from build123d import *

# Parameters (mm, degrees)
F_3_8_0_375_DIAMETER_HOLE1_D     = 9.525
F_3_8_0_375_DIAMETER_HOLE1_DEPTH = 5.999988
F_3_8_0_375_DIAMETER_HOLE1_TIP   = 2.861598698
SKETCH6_W                        = 0.6
SKETCH6_H                        = 2
BOSS_EXTRUDE1_DEPTH              = 5.5


with BuildPart() as part:
    # Sketch1 → Revolve2 (revolve)
    with BuildSketch(Plane(origin=(0, 0, 0), x_dir=(1, 0, 0), z_dir=(0, 1, 0))):
        Polygon((0, 0), (6.35, 0), (6.35, 17.5), (7.5, 17.5), (7.5, 18.5), (6.5, 19.5), (0, 19.5), align=None)
    revolve(axis=Axis((0, 0, -19.5), (0, 0, 1)))

    # 3/8 (0.375) Diameter Hole1
    with Locations(Plane(origin=(0, 0, -19.5), x_dir=(-1, 0, 0), z_dir=(0, 0, -1))):
        with Locations((0, 0)):
            Hole(F_3_8_0_375_DIAMETER_HOLE1_D / 2, depth=F_3_8_0_375_DIAMETER_HOLE1_DEPTH)
            with Locations((0, 0, -(F_3_8_0_375_DIAMETER_HOLE1_DEPTH + F_3_8_0_375_DIAMETER_HOLE1_TIP / 2))):  # 118° drill point
                Cone(0, F_3_8_0_375_DIAMETER_HOLE1_D / 2, F_3_8_0_375_DIAMETER_HOLE1_TIP, mode=Mode.SUBTRACT)

    # Sketch6 → Boss-Extrude1 (add)
    with BuildSketch(Plane.XY):
        with Locations((-3, 0)):
            Rectangle(SKETCH6_W, SKETCH6_H)
    boss_extrude1 = extrude(amount=BOSS_EXTRUDE1_DEPTH)

    # Mirror1: Boss-Extrude1 across plane
    add(boss_extrude1.mirror(Plane(origin=(0, 0, 0), x_dir=(0, 0, 1), z_dir=(1, 0, 0))))


solid = part.part
Verification items for the finished model (mm, model axes). A direction names the side the tool comes from. Coordinates: 2 decimals unless noted, no trailing zeros. Write each loop counter-clockwise with the first axis right and the second up, starting at its lowest first coordinate (ties: lowest second). Pieces come first, ordered by that corner, then holes. Notation, with made-up numbers: M 5,-39 L 51,-39 A20 cw 51,-33 Z; hole C 39,70 d4. An arc over 180 degrees is marked long. One line per question, with ' | ' between items.
1) Release check for a two-part mould opening along X. For faces 4 (the face through (-1.38, -6.2, -8.87)), 5 (the face through (2.7, 0, 3)), 6 (the face through (-3.78, -2.9, -16.46)), 7 (the face through (-3.3, 0, 3)) record: +X half, -X half, draft (parallel to the pull), parting line (faces both ways), or undercut.
Solutions:
face 4: parting line | face 5: undercut | face 6: undercut | face 7: -X half
2) Material ranges on L1, parallel to Y at x = 0, z = -16.75; L2, parallel to Y at x = 0, z = -17.85; L3, parallel to X at y = 0.75, z = 1.5, recorded low to high.
Solutions:
L1: -6.35 to -4.76, 4.76 to 6.35 | L2: -7.5 to -4.76, 4.76 to 7.5 | L3: -3.3 to -2.7, 2.7 to 3.3
3) Depth check by flat-ended pin: pin 1 Ø5 at (y, z) = (0, 3) entering from -X; pin 2 Ø1 at (y, z) = (-2, -7) entering from -X; pin 3 Ø1 at (y, z) = (-0.5, 3.5) entering from +X. Enter the tip coordinate at first touch or a pass-through.
Solutions:
pin 1: x = -3.3 | pin 2: x = -6.17 | pin 3: x = 3.3
4) Sectioned sample at A-A on z = 3.5. Record the cut outline in (x, y).
Solutions:
outline: M -3.3,-1 L -2.7,-1 L -2.7,1 L -3.3,1 Z; M 2.7,-1 L 3.3,-1 L 3.3,1 L 2.7,1 Z
5) Sectioned sample at C-C on z = -12.75. Record the cut outline in (x, y), then the cut area to 3 significant figures.
Solutions:
outline: C 0,0 d12.7; hole C 0,0 d7.03 | area: 87.9 mm^2
6) Access from +Z, -Z, +X, -X, +Y, -Y to the whole of each face (thin tool, end or side, straight path). Record for faces 1 (the face through (3.3, 0, 3)), 2 (the face through (6, 3, -17.5)), 3 (the face through (-2.7, 0, 3)).
Solutions:
face 1: +Z, +X, +Y, -Y | face 2: +Z | face 3: +Z, +Y, -Y
7) Sectioned sample at B-B on z = -8.75. Record the cut outline in (x, y).
Solutions:
outline: C 0,0 d12.7
